Geometry check sheet. Reference: drawing and pictorial views, mm from the part's lowest x, y, z. A direction names the side the tool comes from. Give positions to 0.01 mm unless a question says otherwise; leave off trailing zeros. Write each loop counter-clockwise with the first axis right and the second up, starting at its lowest first coordinate (ties: lowest second). Pieces come first, ordered by that corner, then holes. Notation, with made-up numbers: M 9,5 L 29,5 A35 ccw 29,44 Z; hole C -12.75,31 d7. An arc over 180 degrees is marked long. One line per item, written item: value. Start each with the question number.
1. Scan lines: line 1 (Z direction, x = 65, y = 20.6); line 2 (X direction, y = 15.5, z = 24.25); line 3 (Z direction, x = 5, y = 20.5). Record each from-to range of solid material in increasing order.
2. Gauge pin test, flat ends, axial feed: pin 1 (5 mm diameter, centred on y = 17.5, z = 21, fed in from -X); pin 2 (1.1 mm diameter, centred on y = 20.5, z = 11.5, fed in from +X); pin 3 (6 mm diameter, centred on x = 55, z = 15, fed in from +Y); pin 4 (1.1 mm diameter, centred on y = 20.5, z = 20, fed in from -X). Record the tip position at first contact, or that the pin passes through.
3. Cross-section at D-D on z = 15. Count the separate pieces of the cut face and the enclosed holes in it.
4. Release check for a two-part mould opening along X. For the marked faces 1, 2, 3 and 4 record: pulls with the +X half, pulls with the -X half, needs draft (parallel to the pull), parting line crosses it, or undercut.
5. Tool access check on the marked faces 5 and 6. Record the directions out of +Z, -Z, +X, -X, +Y, -Y that give a thin tool (end or side, any length) a straight path to the whole face; none if there is none.
6. Cross-section at C-C on z = 5. Record the cut outline in (x, y).
7. Cross-section at A-A on y = 7.25. Record the cut outline in (x, z).
8. Cross-section at B-B on x = 15. Record the cut outline in (y, z), then the cut area to 3 significant figures.
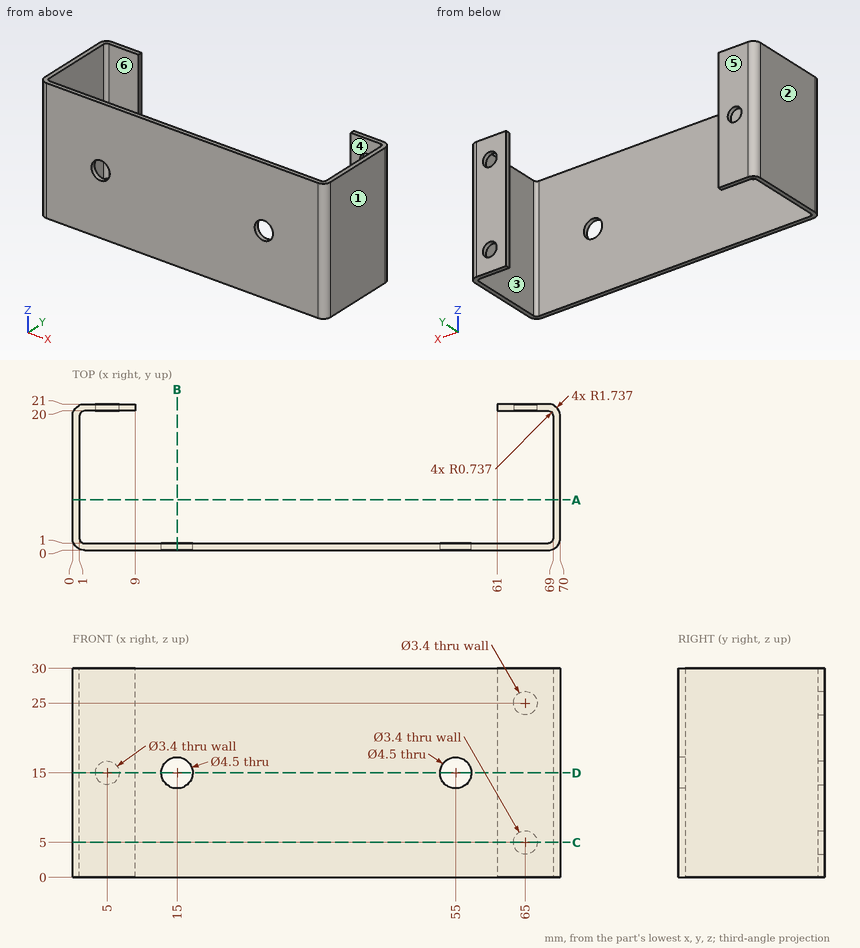
Report:
1. line 1: z = 0 to 3.3, 6.7 to 23.3, 26.7 to 30
1. line 2: x = 0 to 1, 69 to 70
1. line 3: z = 0 to 13.3, 16.7 to 30
2. pin 1: stops at x = 0
2. pin 2: stops at x = 69.86
2. pin 3: stops at y = 1
2. pin 4: stops at x = 0.14
3. separate pieces: 4
3. enclosed holes: 0
4. face 1: pulls with the +X half
4. face 2: pulls with the -X half
4. face 3: undercut
4. face 4: undercut
5. face 5: +Z, -Z, +X, -X, +Y
5. face 6: +Z, -Z
6. outline: M 0,1.74 A1.74 ccw 1.74,0 L 68.26,0 A1.74 ccw 70,1.74 L 70,19.26 A1.74 ccw 68.26,21 L 66.7,21 L 66.7,20 L 68.26,20 A0.74 cw 69,19.26 L 69,1.74 A0.74 cw 68.26,1 L 1.74,1 A0.74 cw 1,1.74 L 1,19.26 A0.74 cw 1.74,20 L 9,20 L 9,21 L 1.74,21 A1.74 ccw 0,19.26 Z; M 61,20 L 63.3,20 L 63.3,21 L 61,21 Z
7. outline: M 0,0 L 1,0 L 1,30 L 0,30 Z; M 69,0 L 70,0 L 70,30 L 69,30 Z
8. outline: M 0,0 L 1,0 L 1,12.75 L 0,12.75 Z; M 0,17.25 L 1,17.25 L 1,30 L 0,30 Z
8. area: 25.5 mm^2
